Can you work these out from the model? Positions are in its coordinate system, mm. Face numbers are marked on the shaded views. A direction names the side the tool comes from. Coordinates: 2 decimals unless noted, no trailing zeros. Order: outer loops, then holes, each group sorted by start corner. A loop starts at its lowest first (then second) coordinate and runs counter-clockwise, first axis right, second up.
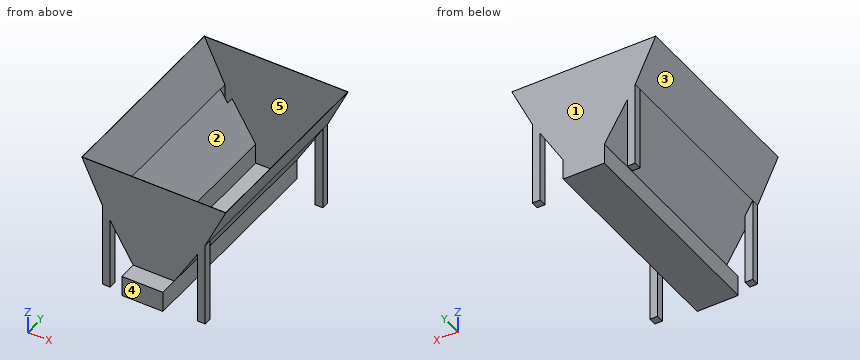
```python
from build123d import *

# Parameters (mm, degrees)
F1_DEPTH = 1930.4
F3_W     = 76.2
F3_H     = 76.2
F5_W     = 406.4
F5_H     = 203.2
F6_DEPTH = 180.34
F7_T     = -2.54


with BuildPart() as f1:
    # F0 (on Front) → F1 (new body)
    with BuildSketch(Plane.XZ):
        Polygon((-203.2, 0), (0, 0), (203.2, 0), (203.2, 203.2), (508, 711.2), (711.2, 1143), (0, 1143), (-711.2, 1143), (-508, 711.2), (-203.2, 203.2), align=None)
    extrude(amount=F1_DEPTH)

    # F3 (on offset) → F4 (join, up to the next surface of F1)
    with BuildSketch(Plane(origin=(0, 0, -127), x_dir=(1, 0, 0), z_dir=(0, 0, -1))):
        with Locations((-469.9, 1892.3)):
            Rectangle(F3_W, F3_H)
        with Locations((469.9, 1892.3)):
            Rectangle(F3_W, F3_H)
        with Locations((469.9, 38.1)):
            Rectangle(F3_W, F3_H)
        with Locations((-469.9, 38.1)):
            Rectangle(F3_W, F3_H)
    extrude(until=Until.NEXT, dir=(0, 0, 1))

    # F5 (on face) → F6 (join)
    with BuildSketch(Plane.XZ.offset(1930.4)):
        with Locations((0, 101.6)):
            Rectangle(F5_W, F5_H)
    extrude(amount=F6_DEPTH)

    # F7
    f7_openings = [f1.faces().sort_by_distance(p)[0] for p in [
        (0, -965.2, 1143),
    ]]
    offset(amount=F7_T, openings=f7_openings, kind=Kind.INTERSECTION)


solid = f1.part
```
1. Thinking about a two-plate mould opening in X: for the marked faces 3, 4 and 5, which applies, pulls with the +X half, pulls with the -X half, needs draft (parallel to the pull), parting line crosses it, or undercut?
Completed:
face 3: pulls with the -X half
face 4: needs draft
face 5: undercut
2. Imagine slicing it at A-A on y = -938.5. Please give me the cut outline in (x, z), then the cut area to 3 significant figures.
Completed:
outline: (-711.2, 1143) - (-508, 711.2) - (-203.2, 203.2) - (-203.2, 0) - (203.2, 0) - (203.2, 203.2) - (508, 711.2) - (711.2, 1143) - (708.39, 1143) - (505.76, 712.4) - (200.66, 203.9) - (200.66, 2.54) - (-200.66, 2.54) - (-200.66, 203.9) - (-505.76, 712.4) - (-708.39, 1143) - close
area: 7,490 mm2
3. On a 3-axis mill with a long thin cutter (end or side, diameter ignored), from which of +Z, -Z, +X, -X, +Y, -Y can I reach the whole of each face in a straight line? I mean the marked faces 1 and 2. Say none if no direction works.
Completed:
face 1: +Z, -Z, +X, -X, +Y
face 2: +Z
4. Please list where these lines run through material, in increasing order: probe 1 along Y at (x, z) = (267.5, 768.5); probe 2 along Y at (x, z) = (454.5, 472); probe 3 along Y at (x, z) = (135, 69.5).
Completed:
probe 1: y = -1930.4 to -1927.86, -2.54 to 0
probe 2: y = -1930.4 to -1927.86, -1856.74 to -1854.2, -76.2 to -73.66, -2.54 to 0
probe 3: y = -2110.74 to -2108.2, -2.54 to 0
5. I'm going to push flat-ended pins straight in: pin 1 (10 mm diameter, centred on x = -19, y = -1056.5, fed in from -Z); pin 2 (1.5 mm diameter, centred on x = -546.5, y = -399, fed in from -Z); pin 3 (12 mm diameter, centred on x = 299, y = -1055, fed in from +Z). Where does each tip first touch, or does it pass through?
Completed:
pin 1: stops at z = 0
pin 2: stops at z = 791.42
pin 3: stops at z = 377.8
6. Imagine slicing it at C-C on z = 146.5. Give the number of separate pieces and of enclosed holes in the cut face, then the cut area to 3 significant figures.
Completed:
separate pieces: 5
enclosed holes: 5
area: 15,800 mm2
7. Imagine slicing it at B-B on x = -136. Please give me the cut outline in (y, z).
Completed:
outline: (-2110.74, 0) - (0, 0) - (0, 1143) - (-2.54, 1143) - (-2.54, 2.54) - (-2108.2, 2.54) - (-2108.2, 200.66) - (-1927.86, 200.66) - (-1927.86, 1143) - (-1930.4, 1143) - (-1930.4, 203.2) - (-2110.74, 203.2) - close
